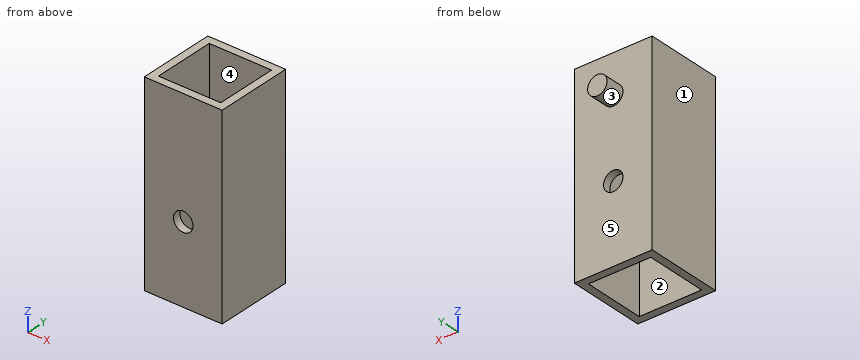
```python
from build123d import *

# Parameters (mm, degrees)
SKETCH1_W           = 25.4
SKETCH1_H           = 25.4
SKETCH1_W_2         = 20.32
SKETCH1_H_2         = 20.32
EXTRUDE_THIN1_DEPTH = 31.75
SKETCH2_R           = 3.175
BOSS_EXTRUDE1_DEPTH = 6.35
SKETCH4_R           = 3.175
CUT_EXTRUDE1_DEPTH  = 26.4


with BuildPart() as part:
    # Sketch1 → Extrude-Thin1 (new body, symmetric)
    with BuildSketch(Plane.XY):
        Rectangle(SKETCH1_W, SKETCH1_H)
        Rectangle(SKETCH1_W_2, SKETCH1_H_2, mode=Mode.SUBTRACT)
    extrude(amount=EXTRUDE_THIN1_DEPTH, both=True)

    # Sketch2 → Boss-Extrude1 (add)
    with BuildSketch(Plane(origin=(0, 12.7, 0), x_dir=(1, 0, 0), z_dir=(0, 1, 0))):
        with Locations((0, -19.05)):
            Circle(SKETCH2_R)
    extrude(amount=BOSS_EXTRUDE1_DEPTH)

    # Sketch4 → Cut-Extrude1 (cut, through all)
    with BuildSketch(Plane(origin=(0, 12.7, 0), x_dir=(1, 0, 0), z_dir=(0, 1, 0))):
        with Locations((0, 6.35)):
            Circle(SKETCH4_R)
    extrude(amount=-CUT_EXTRUDE1_DEPTH, mode=Mode.SUBTRACT)


solid = part.part
```
Geometry: final body of the model. Coordinates: model frame, mm. Face numbers are marked on the shaded views. A direction names the side the tool comes from. Round coordinates to 2 decimals unless told otherwise and drop trailing zeros. Order: outer loops, then holes, each group sorted by start corner. A loop starts at its lowest first (then second) coordinate and runs counter-clockwise, first axis right, second up. Notation, with made-up numbers: (-39.5, -21.75) - (15.5, -21.75) arc R33 ccw to (15.5, 15.25) - close; hole circle Ø4 at (58.25, 84.5). An arc over 180 degrees is marked (long way). Use CSV: the item, a comma, the result in double quotes. Start each with the question number.
Q1. Mould query, pull axis X, two halves, no side actions, for the marked faces 3, 4 and 5. Classes: +X half, -X half, draft (parallel to the pull), parting line (faces both ways), or undercut.
Q2. Section query A-A (x = -4). Return loops of the section in (y, z).
Q3. Access query for the marked faces 1 and 2. Directions: +Z, -Z, +X, -X, +Y, -Y. A direction counts if a zero-diameter tool reaches every point of the face in a straight line with its end or side. Return the directions, or none.
Q4. Material intervals for line 1 along X through (y, z) = (11.3, -6.35) (3 decimals); line 2 along Z through (x, y) = (0, -10.7) (3 decimals); line 3 along Y through (x, z) = (10, 8), sorted ascending. Write a range as from..to.
Q5. Section query D-D (x = 1). Return loops of the section in (y, z), and give its area (3 significant figures).
Q6. First-contact query: pin 1 (8 mm diameter, centred on x = 4, y = 6.5, fed in from +Z); pin 2 (7.5 mm diameter, centred on x = -0.5, z = 4, fed in from +Y); pin 3 (4 mm diameter, centred on x = 2.5, y = -7, fed in from +Z). Flat tips, straight axial feed; report the tip coordinate or a pass-through.
Q7. Section query B-B (z = -21). Return loops of the section in (x, y).
Result set:
1,face 3,"parting line"
1,face 4,"undercut"
1,face 5,"draft"
2,outline,"(-12.7, -31.75) - (-10.16, -31.75) - (-10.16, 31.75) - (-12.7, 31.75) - close; (10.16, -31.75) - (12.7, -31.75) - (12.7, 31.75) - (10.16, 31.75) - close"
3,face 1,"+Z, -Z, -X, +Y, -Y"
3,face 2,"+Z, -Z"
4,line 1,"x = -12.7..-3.175, 3.175..12.7"
4,line 2,"z = -31.75..-9.525, -3.175..31.75"
4,line 3,"y = -12.7..-10.16, 10.16..12.7"
5,outline,"(-12.7, -31.75) - (-10.16, -31.75) - (-10.16, -9.36) - (-12.7, -9.36) - close; (-12.7, -3.34) - (-10.16, -3.34) - (-10.16, 31.75) - (-12.7, 31.75) - close; (10.16, -31.75) - (12.7, -31.75) - (12.7, -9.36) - (10.16, -9.36) - close; (10.16, -3.34) - (12.7, -3.34) - (12.7, 16.04) - (19.05, 16.04) - (19.05, 22.06) - (12.7, 22.06) - (12.7, 31.75) - (10.16, 31.75) - close"
5,area,"330 mm2"
6,pin 1,"stops at z = 31.75"
6,pin 2,"stops at y = 12.7"
6,pin 3,"passes through"
7,outline,"(-12.7, -12.7) - (12.7, -12.7) - (12.7, 12.7) - (-12.7, 12.7) - close; hole (-10.16, -10.16) - (10.16, -10.16) - (10.16, 10.16) - (-10.16, 10.16) - close"
